The drawing under review shows one solid part. Ordinate dimensions are in mm from its lowest x, y, z. Round coordinates to 2 decimals unless told otherwise and drop trailing zeros. Write each loop counter-clockwise with the first axis right and the second up, starting at its lowest first coordinate (ties: lowest second). Pieces come first, ordered by that corner, then holes. Notation, with made-up numbers: (77.25, 36.25) - (130.25, 36.25) arc R20 ccw to (130.25, 46.25) - close; hole circle Ø2 at (61.5, 21). An arc over 180 degrees is marked (long way). One line per question, with ' | ' between items. Start each with the question number.
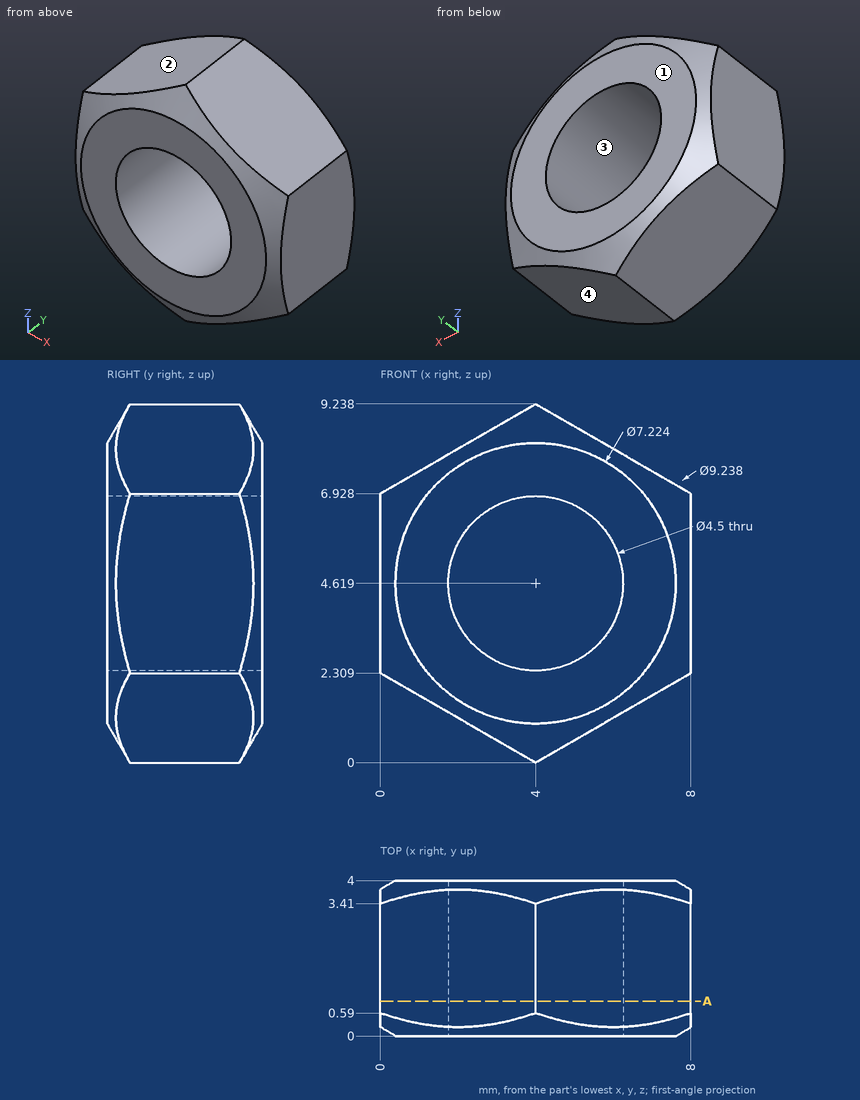
1. The part is to be moulded in two halves that separate along Z. For the marked faces 1, 2, 3 and 4, say which applies: pulls with the +Z half, pulls with the -Z half, needs draft (parallel to the pull), parting line crosses it, or undercut.
2. Clearance check with a flat-ended pin moving along its axis: P1, Ø1.5, axis at x = 6, y = 3, coming from the +Z side (1 decimal). State where the tip first meets the part, or that it passes through.
3. Add section A-A, the plane y = 0.9. Write out the cut boundary in (x, z).
4. Wall thickness on line 1 along X through (y, z) = (1.55, 5); line 2 along X through (y, z) = (2.3, 5.5); line 3 along Z through (x, y) = (2.5, 1.1) (1 decimal): over which ranges is each line inside the solid? List them lowest first. Write a range as [from, to].
Geometry check:
1) face 1: needs draft | face 2: pulls with the +Z half | face 3: undercut | face 4: pulls with the -Z half
2) P1: stops at z = 8.5
3) outline: (0, 2.31) - (4, 0) - (8, 2.31) - (8, 6.93) - (4, 9.24) - (0, 6.93) - close; hole circle Ø4.5 at (4, 4.62)
4) line 1: x = [0, 1.78], [6.22, 8] | line 2: x = [0, 1.93], [6.07, 8] | line 3: z = [0.9, 2.9], [6.3, 8.4]
